from build123d import *

# Parameters (mm, degrees)
SKETCH002_W     = 126
SKETCH002_H     = 16
PAD001_DEPTH    = 16
SKETCH003_W     = 120.5
SKETCH003_H     = 10.5
POCKET001_DEPTH = 12.64
FILLET001_R     = 3.25
FILLET003_R     = 3.4


with BuildPart() as obj1:
    # Sketch002 → Pad001 (new body)
    with BuildSketch(Plane.XY):
        Rectangle(SKETCH002_W, SKETCH002_H)
    extrude(amount=PAD001_DEPTH)

    # Sketch003 (on DatumPlane) → Pocket001 (cut)
    with BuildSketch(Plane.XY.offset(16)):
        Rectangle(SKETCH003_W, SKETCH003_H)
    extrude(amount=-POCKET001_DEPTH, mode=Mode.SUBTRACT)

    # Fillet001
    fillet001_edges = [obj1.edges().sort_by_distance(p)[0] for p in [
        (-60.25, 5.25, 9.68),
        (-60.25, -5.25, 9.68),
        (60.25, -5.25, 9.68),
        (60.25, 5.25, 9.68),
    ]]
    fillet(fillet001_edges, radius=FILLET001_R)


with BuildPart() as fillet003:
    # Body001003 base: copy of obj1
    add(obj1.part)


with BuildPart() as fillet003_1:
    # Body001003 placement: moved
    add(fillet003.part.moved(Location((0, -16, 0))))

    # Fillet003
    fillet003_edges = [fillet003_1.edges().sort_by_distance(p)[0] for p in [
        (-63, -24, 8),
        (63, -24, 8),
    ]]
    fillet(fillet003_edges, radius=FILLET003_R)


with BuildPart() as obj2:
    # Fusion base: copy of obj1
    add(obj1.part)

    # Fusion: union Fillet003
    add(fillet003_1.part)


solid = obj2.part
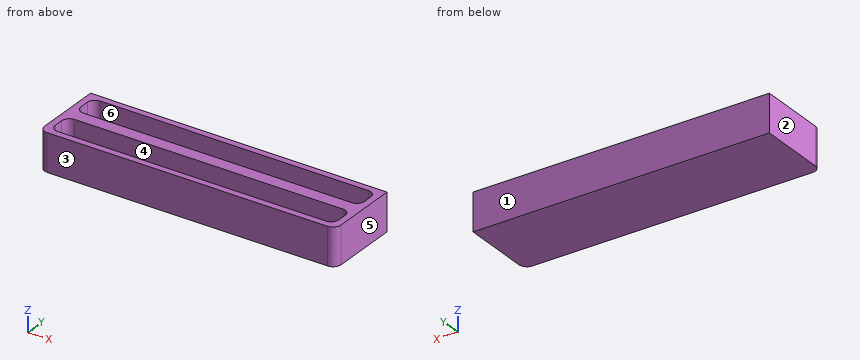
Build history of the part. All positions in model axes, mm. Face numbers are marked on the shaded views. A direction names the side the tool comes from. Coordinates: 2 decimals unless noted, no trailing zeros. Order: outer loops, then holes, each group sorted by start corner. A loop starts at its lowest first (then second) coordinate and runs counter-clockwise, first axis right, second up. Notation, with made-up numbers: (-5.5, 88) - (51.5, 88) arc R7 cw to (51.5, 93) - close; hole circle Ø11 at (44, 44.5). An arc over 180 degrees is marked (long way). Write each question's results on one line, items separated by ' | '. Start each with the question number.
Item 1: Wall check: probe 1 along Y at (x, z) = (-3.5, 6.5); probe 2 along X at (y, z) = (-17, 3.75); probe 3 along Z at (x, y) = (-7, 1.5). Give the ranges that are in metal, low to high. Write a range as [from, to].
Item 2: Band-saw the part on A-A on z = 7.5. Write the cut outline in (x, y).
Item 3: Band-saw the part on C-C on x = 4. Write the cut outline in (y, z).
Item 4: Mould opens along Y. For the marked faces 1, 2, 3 and 4 say: released by +Y, released by -Y, zero draft, split by the parting line, or undercut.
Item 5: Band-saw the part on B-B on y = -16.5. Write the cut outline in (x, z).
Item 6: Tool access for the marked faces 5 and 6: list every direction of +Z, -Z, +X, -X, +Y, -Y with a clear straight run to the whole face (end or side of a thin tool).
Numbers:
1) probe 1: [-24, -21.25], [-10.75, -5.25], [5.25, 8] | probe 2: [-63, -60.25], [60.25, 63] | probe 3: [0, 3.36]
2) outline: (-63, -20.6) arc R3.4 ccw to (-59.6, -24) - (59.6, -24) arc R3.4 ccw to (63, -20.6) - (63, 8) - (-63, 8) - close; hole (-60.25, -18) arc R3.25 ccw to (-57, -21.25) - (57, -21.25) arc R3.25 ccw to (60.25, -18) - (60.25, -14) arc R3.25 ccw to (57, -10.75) - (-57, -10.75) arc R3.25 ccw to (-60.25, -14) - close; hole (-60.25, -2) arc R3.25 ccw to (-57, -5.25) - (57, -5.25) arc R3.25 ccw to (60.25, -2) - (60.25, 2) arc R3.25 ccw to (57, 5.25) - (-57, 5.25) arc R3.25 ccw to (-60.25, 2) - close
3) outline: (-24, 0) - (8, 0) - (8, 16) - (5.25, 16) - (5.25, 3.36) - (-5.25, 3.36) - (-5.25, 16) - (-10.75, 16) - (-10.75, 3.36) - (-21.25, 3.36) - (-21.25, 16) - (-24, 16) - close
4) face 1: released by +Y | face 2: zero draft | face 3: released by -Y | face 4: undercut
5) outline: (-63, 0) - (63, 0) - (63, 16) - (60.25, 16) - (60.25, 3.36) - (-60.25, 3.36) - (-60.25, 16) - (-63, 16) - close
6) face 5: +Z, -Z, +X, +Y, -Y | face 6: +Z
